For this review, use the dimensioned drawing (mm, ordinates from the lowest corner) and the shaded views. Round coordinates to 2 decimals unless told otherwise and drop trailing zeros. Write each loop counter-clockwise with the first axis right and the second up, starting at its lowest first coordinate (ties: lowest second). Pieces come first, ordered by that corner, then holes. Notation, with made-up numbers: (-18.75, 19) -> (40.25, 19) arc R34 cw to (40.25, 53) -> close; hole circle Ø5 at (80, 45). An arc over 180 degrees is marked (long way). Write each question's results on one line, items separated by ' | '. Start each with the question number.
Item 1: Add section D-D (z = 2.9). State the section outline as (x, y) points, plus the area to 3 significant figures.
Item 2: Add section C-C (x = 76.9). State the section outline as (y, z) points, plus the area to 3 significant figures.
Item 3: To check wall thickness, follow line 1 along Z through (x, y) = (53.5, 0.45); line 2 along Z through (x, y) = (31, 1.75); line 3 along X through (y, z) = (1.3, 7). State the ranges of each line that lie inside material, in increasing order.
Item 4: Clearance check with flat-ended pins moving along their axes: pin 1 (1 mm diameter, centred on x = 29.5, y = 0.5, fed in from -Z); pin 2 (10 mm diameter, centred on x = 12.5, z = 49.5, fed in from +Y); pin 3 (2 mm diameter, centred on y = 1, z = 29.5, fed in from +X). State where each tip first meets the part, or that it passes through.
Item 5: Add section A-A (z = 17.5). State the section outline as (x, y) points, plus the area to 3 significant figures.
Item 6: Add section B-B (y = 0.9). State the section outline as (x, z) points.
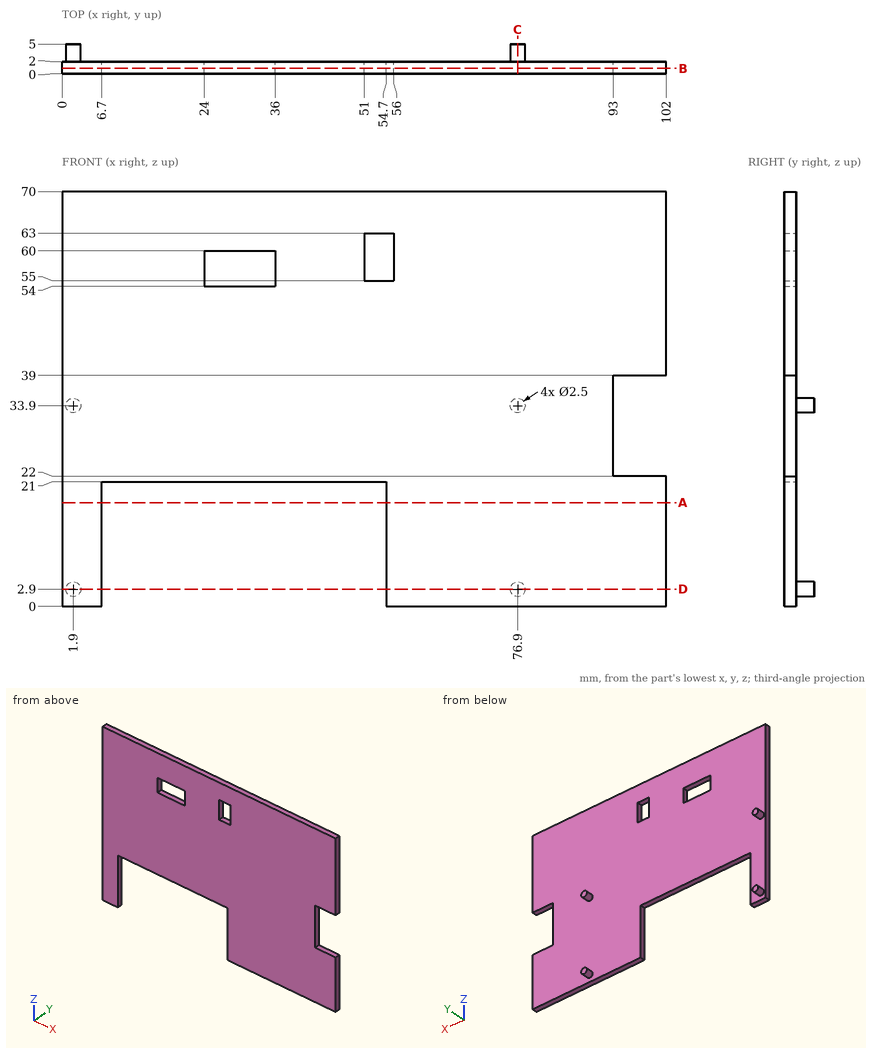
Responses:
1) outline: (0, 0) -> (6.7, 0) -> (6.7, 2) -> (3.15, 2) -> (3.15, 5) -> (0.65, 5) -> (0.65, 2) -> (0, 2) -> close; (54.7, 0) -> (102, 0) -> (102, 2) -> (78.15, 2) -> (78.15, 5) -> (75.65, 5) -> (75.65, 2) -> (54.7, 2) -> close | area: 123 mm^2
2) outline: (0, 0) -> (2, 0) -> (2, 1.65) -> (5, 1.65) -> (5, 4.15) -> (2, 4.15) -> (2, 32.65) -> (5, 32.65) -> (5, 35.15) -> (2, 35.15) -> (2, 70) -> (0, 70) -> close | area: 155 mm^2
3) line 1: z = 21 to 55, 63 to 70 | line 2: z = 21 to 54, 60 to 70 | line 3: x = 0 to 6.7, 54.7 to 102
4) pin 1: stops at z = 21 | pin 2: stops at y = 2 | pin 3: stops at x = 93
5) outline: (0, 0) -> (6.7, 0) -> (6.7, 2) -> (0, 2) -> close; (54.7, 0) -> (102, 0) -> (102, 2) -> (54.7, 2) -> close | area: 108 mm^2
6) outline: (0, 0) -> (6.7, 0) -> (6.7, 21) -> (54.7, 21) -> (54.7, 0) -> (102, 0) -> (102, 22) -> (93, 22) -> (93, 39) -> (102, 39) -> (102, 70) -> (0, 70) -> close; hole (24, 54) -> (36, 54) -> (36, 60) -> (24, 60) -> close; hole (51, 55) -> (56, 55) -> (56, 63) -> (51, 63) -> close
